Could you check a few things on this drawing? It's one solid part, dimensions in mm from its lowest x, y, z. A direction names the side the tool comes from. Coordinates: 2 decimals unless noted, no trailing zeros. Order: outer loops, then holes, each group sorted by start corner. A loop starts at its lowest first (then second) coordinate and runs counter-clockwise, first axis right, second up. Notation, with made-up numbers: (-25.5, 24.25) - (-20.5, 24.25) arc R14 cw to (-20.5, 46.25) - close; hole circle Ø6 at (17.25, -25). An arc over 180 degrees is marked (long way). Answer in a Markdown table with one row per item. Add a question column.
Item 1: If I drill on line 1 along Z through (x, y) = (18, 57) (1 decimal); line 2 along X through (y, z) = (51.5, 65) (1 decimal); line 3 along X through (y, z) = (26.5, 66), over which ranges is the centre line in solid material (lowest first)? Write a range as from..to.
Item 2: I want a section at C-C (z = 54). Please give me the cut outline in (x, y) (1 decimal).
Item 3: I want a section at A-A (x = 31). Please give me the cut outline in (y, z) (1 decimal).
Item 4: Thinking about a two-plate mould opening in X: for the marked faces 1, 2 and 3, which applies, +X half, -X half, draft (parallel to the pull), parting line (faces both ways), or undercut?
Item 5: I want a section at B-B (y = 8). Please give me the cut outline in (x, z) (1 decimal).
Item 6: On a 3-axis mill with a long thin cutter (end or side, diameter ignored), from which of +Z, -Z, +X, -X, +Y, -Y can I reach the whole of each face in a straight line? I mean the marked faces 4 and 5. Say none if no direction works.
Item 7: Will these pins go through, and if not, where does the flat tip stop? pin 1 Ø1 at (y, z) = (60, 10.5) entering from +X; pin 2 Ø5 at (y, z) = (20, 23) entering from +X.
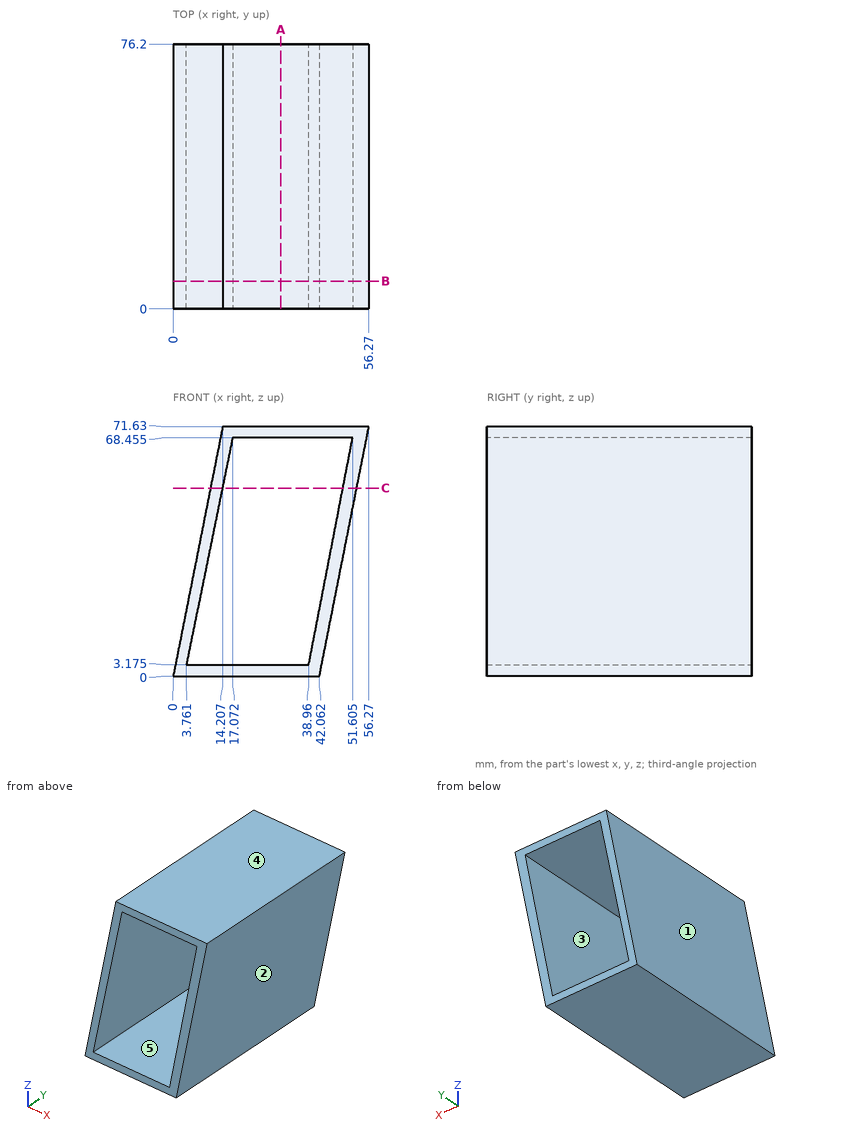
Values follow:
| question | item | result |
|---|---|---|
| 1 | line 1 | z = 0..3.2, 68.5..71.6 |
| 1 | line 2 | x = 12.9..16.4, 50.9..55 |
| 1 | line 3 | x = 13.09..16.57, 51.13..55.15 |
| 2 | outline | (10.7, 0) - (14.1, 0) - (14.1, 76.2) - (10.7, 76.2) - close; (48.8, 0) - (52.8, 0) - (52.8, 76.2) - (48.8, 76.2) - close |
| 3 | outline | (0, 0) - (76.2, 0) - (76.2, 3.2) - (0, 3.2) - close; (0, 68.5) - (76.2, 68.5) - (76.2, 71.6) - (0, 71.6) - close |
| 4 | face 1 | -X half |
| 4 | face 2 | +X half |
| 4 | face 3 | undercut |
| 5 | outline | (0, 0) - (42.1, 0) - (56.3, 71.6) - (14.2, 71.6) - close; hole (3.8, 3.2) - (39, 3.2) - (51.6, 68.5) - (17.1, 68.5) - close |
| 6 | face 4 | +Z, +X, -X, +Y, -Y |
| 6 | face 5 | +Y, -Y |
| 7 | pin 1 | stops at x = 44.24 |
| 7 | pin 2 | stops at x = 47.12 |
